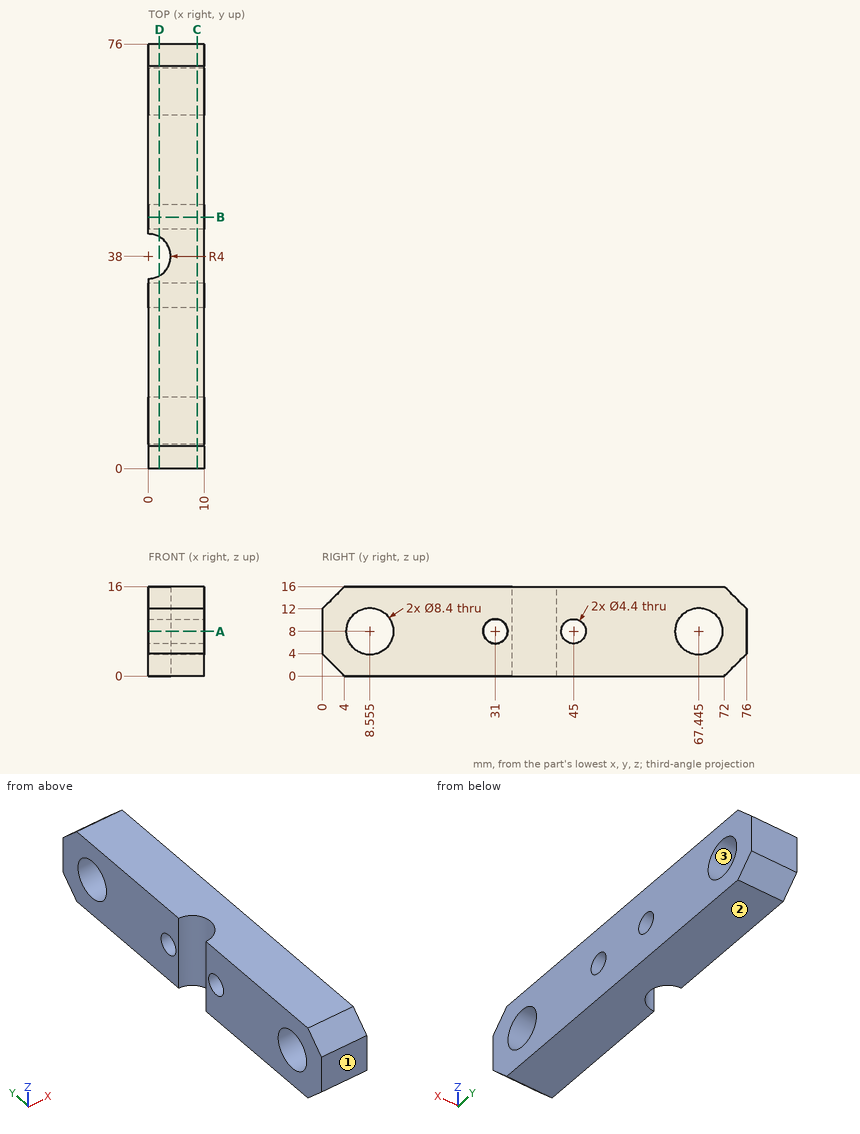
Verification items for this drawing (mm, ordinates from the low corner). Give positions to 0.01 mm unless a question says otherwise; leave off trailing zeros. Loops run counter-clockwise (first coordinate to the right, second up) from the corner with the lowest first, then second, coordinate; pieces in that order, holes last. Notation, with made-up numbers: M 32,-1 L 52,-1 A8 ccw 52,8 Z; hole C -9,59 d6. An arc over 180 degrees is marked long. Return JSON: item names as keys, results as strings. Group by question number.
1. Cross-section at B-B on y = 45. Record the boundary of the cut face in (x, z), plus the area to 3 significant figures.
2. Cross-section at C-C on x = 8.75. Record the boundary of the cut face in (y, z) (3 decimals), plus the area to 3 significant figures.
3. Mould release check, pull along Z, two halves, no side actions. Record for the marked faces 1, 2 and 3: released by +Z, released by -Z, zero draft, split by the parting line, or undercut.
4. Cross-section at D-D on x = 2. Record the boundary of the cut face in (y, z) (3 decimals).
5. Cross-section at A-A on z = 8. Record the boundary of the cut face in (x, y) (3 decimals).
6. Thickness scan on L1, parallel to Y at x = 7, z = 8 (3 decimals); L2, parallel to Z at x = 6, y = 31; L3, parallel to Y at x = 9.25, z = 7. Record the ranges inside material, lowest first.
Return value:
{
 "1": {"outline": "M 0,0 L 10,0 L 10,5.8 L 0,5.8 Z; M 0,10.2 L 10,10.2 L 10,16 L 0,16 Z", "area": "116 mm^2"},
 "2": {"outline": "M 0,4 L 4,0 L 72,0 L 76,4 L 76,12 L 72,16 L 4,16 L 0,12 Z; hole C 8.555,8 d8.4; hole C 31,8 d4.4; hole C 45,8 d4.4; hole C 67.445,8 d8.4", "area": "1,040 mm^2"},
 "3": {"face 1": "zero draft", "face 2": "released by -Z", "face 3": "undercut"},
 "4": {"outline": "M 0,4 L 4,0 L 34.536,0 L 34.536,16 L 4,16 L 0,12 Z; M 41.464,0 L 72,0 L 76,4 L 76,12 L 72,16 L 41.464,16 Z; hole C 8.555,8 d8.4; hole C 31,8 d4.4; hole C 45,8 d4.4; hole C 67.445,8 d8.4"},
 "5": {"outline": "M 0,0 L 10,0 L 10,4.355 L 0,4.355 Z; M 0,12.755 L 10,12.755 L 10,28.8 L 0,28.8 Z; M 0,33.2 L 10,33.2 L 10,42.8 L 0,42.8 L 0,42 A4 cw 0,34 Z; M 0,47.2 L 10,47.2 L 10,63.245 L 0,63.245 Z; M 0,71.645 L 10,71.645 L 10,76 L 0,76 Z"},
 "6": {"L1": "0 to 4.355, 12.755 to 28.8, 33.2 to 42.8, 47.2 to 63.245, 71.645 to 76", "L2": "0 to 5.8, 10.2 to 16", "L3": "0 to 4.48, 12.63 to 29.04, 32.96 to 43.04, 46.96 to 63.37, 71.52 to 76"}
}
